Part model, mm, in its own coordinate system. Face numbers are marked on the shaded views. A direction names the side the tool comes from. Round coordinates to 2 decimals unless told otherwise and drop trailing zeros. Write each loop counter-clockwise with the first axis right and the second up, starting at its lowest first coordinate (ties: lowest second). Pieces come first, ordered by that corner, then holes. Notation, with made-up numbers: M 63,0 L 83,0 A5 cw 83,7 Z; hole C 55.25,-34.5 d1. An arc over 180 degrees is marked long. Use one line per item in the form item = value. Start each with the question number.
Item 1: Which spindle directions (+Z, -Z, +X, -X, +Y, -Y) get a long thin tool onto all of the face, cutting with end or side? Do the marked faces 1, 2, 3 and 4. Say none if no direction does.
Item 2: Flat gauge pins, fed straight in: pin 1 Ø0.8 at (x, z) = (4, 9) entering from -Y; pin 2 Ø5 at (x, y) = (-1, 14.5) entering from -Z; pin 3 Ø1.6 at (x, z) = (4, 9.5) entering from +Y; pin 4 Ø0.5 at (x, z) = (-0.5, 8) entering from -Y. Where does each tip first touch, or does it go through?
Item 3: Cut at C-C, the plane y = 9.5. Give the cut face in (x, z), then the cut area to 4 significant figures.
Item 4: Cut at A-A, the plane y = 21.75. Give the cut face in (x, z), then the cut area to 4 significant figures.
Item 5: Probe L1, parallel to X at y = 25, z = 9.25; L2, parallel to X at y = 2.5, z = 5.5; L3, parallel to X at y = 12, z = 9. List the from-to ranges inside material, lowest first.
Item 6: Cut at D-D, the plane x = 0.5. Give the cut face in (y, z).
Item 7: Mould opens along X. For the marked faces 5, 6 and 7 say: +X half, -X half, draft (parallel to the pull), parting line (faces both ways), or undercut.
Item 8: Cut at B-B, the plane z = 2.5. Give the cut face in (x, y), then the cut area to 4 significant figures.
from build123d import *

# Parameters (mm, degrees)
SKETCH_W        = 30
SKETCH_H        = 25.5
PAD_DEPTH       = 10
SKETCH001_W     = 25.5
SKETCH001_H     = 30
POCKET_DEPTH    = 8.5
SKETCH002_W     = 20
SKETCH002_H     = 13
POCKET001_DEPTH = 5
CHAMFER_SIZE    = 5
SKETCH003_W     = 2
SKETCH003_H     = 7
POCKET002_DEPTH = 5
SKETCH004_W     = 7
SKETCH004_H     = 2.5
PAD001_DEPTH    = 2
CHAMFER001_SIZE = 1.9


with BuildPart() as part:
    # Sketch → Pad (new body)
    with BuildSketch(Plane.XY):
        with Locations((0, 12.75)):
            Rectangle(SKETCH_W, SKETCH_H)
    extrude(amount=PAD_DEPTH)

    # Sketch001 (on Face5 of Pad) → Pocket (cut)
    with BuildSketch(Plane(origin=(0, 0, 0), x_dir=(1, 0, 0), z_dir=(0, 0, -1))):
        with Locations((0, -15)):
            Rectangle(SKETCH001_W, SKETCH001_H)
    extrude(amount=-POCKET_DEPTH, mode=Mode.SUBTRACT)

    # Sketch002 → Pocket001 (cut)
    with BuildSketch(Plane.XY.offset(10)):
        with Locations((0, 6.5)):
            Rectangle(SKETCH002_W, SKETCH002_H)
    extrude(amount=-POCKET001_DEPTH, mode=Mode.SUBTRACT)

    # Chamfer
    chamfer_edges = [part.edges().sort_by_distance(p)[0] for p in [
        (13.875, 0, 0),
        (-13.875, 0, 0),
    ]]
    chamfer(chamfer_edges, length=CHAMFER_SIZE)

    # Sketch003 (on Face7 of Chamfer) → Pocket002 (cut)
    with BuildSketch(Plane.XY.offset(10)):
        with Locations((-4.5, 22)):
            Rectangle(SKETCH003_W, SKETCH003_H)
        with Locations((4.5, 22)):
            Rectangle(SKETCH003_W, SKETCH003_H)
    extrude(amount=-POCKET002_DEPTH, mode=Mode.SUBTRACT)

    # Sketch004 (on Face17 of Pocket002) → Pad001 (join)
    with BuildSketch(Plane(origin=(0, 25.5, 0), x_dir=(-1, 0, 0), z_dir=(0, 1, 0))):
        with Locations((0, 8.75)):
            Rectangle(SKETCH004_W, SKETCH004_H)
    extrude(amount=PAD001_DEPTH)

    # Chamfer001
    chamfer001_edges = [part.edges().sort_by_distance(p)[0] for p in [
        (0, 27.5, 7.5),
    ]]
    chamfer(chamfer001_edges, length=CHAMFER001_SIZE)


solid = part.part
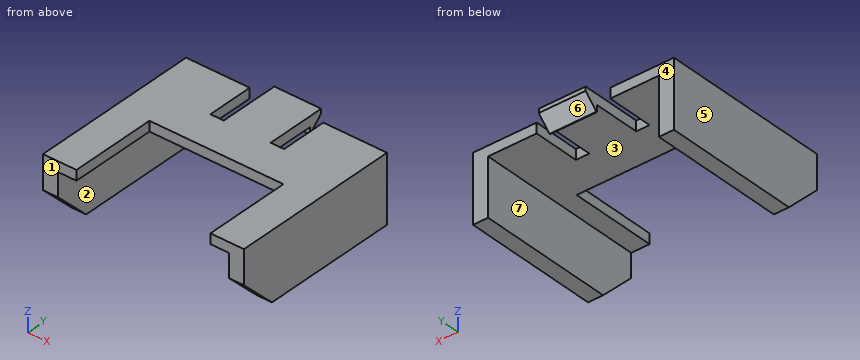
Model answer:
q1.face_1 = +Z, -Z, +X, -X, -Y
q1.face_2 = -Z, +Y, -Y
q1.face_3 = -Z, -Y
q1.face_4 = +Z, -Z, -X, +Y
q2.pin_1 = 13
q2.pin_2 = 8.5
q2.pin_3 = 27.5
q2.pin_4 = 25.5
q3.outline = M -15,0 L -12.75,0 L -12.75,8.5 L -10,8.5 L -10,10 L -15,10 Z; M 10,8.5 L 12.75,8.5 L 12.75,0 L 15,0 L 15,10 L 10,10 Z
q3.area = 53.25 mm²
q4.outline = M -15,0 L -12.75,0 L -12.75,8.5 L -5.5,8.5 L -5.5,10 L -15,10 Z; M -3.5,8.5 L 3.5,8.5 L 3.5,10 L -3.5,10 Z; M 5.5,8.5 L 12.75,8.5 L 12.75,0 L 15,0 L 15,10 L 5.5,10 Z
q4.area = 77.25 mm²
q5.L1 = -15 to -5.5, -3.5 to 3.5, 5.5 to 15
q5.L2 = -15 to -12.75, 12.75 to 15
q5.L3 = -15 to -10, 10 to 15
q6.outline = M 13,8.5 L 25.5,8.5 L 25.5,7.5 L 25.6,7.5 L 27.5,9.4 L 27.5,10 L 13,10 Z
q7.face_5 = -X half
q7.face_6 = draft
q7.face_7 = undercut
q8.outline = M -15,2.5 L -12.75,2.5 L -12.75,25.5 L -15,25.5 Z; M 12.75,2.5 L 15,2.5 L 15,25.5 L 12.75,25.5 Z
q8.area = 103.5 mm²
